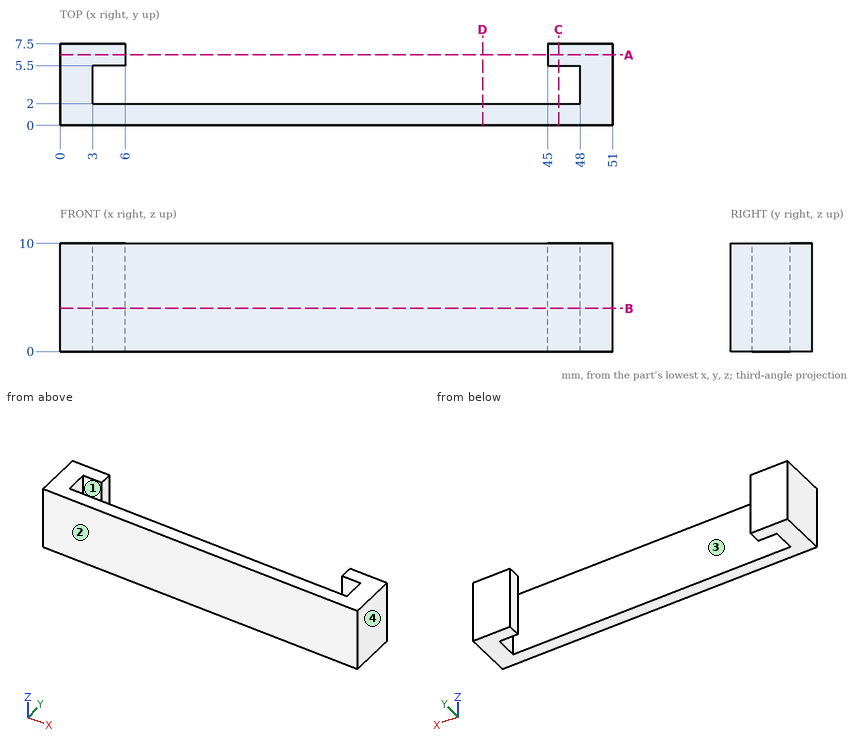
Geometry check sheet. Reference: drawing and pictorial views, mm from the part's lowest x, y, z. Give positions to 0.01 mm unless a question says otherwise; leave off trailing zeros. Order: outer loops, then holes, each group sorted by start corner. A loop starts at its lowest first (then second) coordinate and runs counter-clockwise, first axis right, second up.
1. Thickness scan on L1, parallel to X at y = 3.5, z = 1.25; L2, parallel to Y at x = 46, z = 6.5; L3, parallel to Y at x = 8, z = 6.25. Record the ranges inside material, lowest first.
2. Section check B-B, the plane z = 4. Enter the section's corners in (x, y), and give its area (3 significant figures).
3. Section check A-A, the plane y = 6.5. Enter the section's corners in (x, z).
4. Release check for a two-part mould opening along X. For the marked faces 1, 2, 3 and 4 record: pulls with the +X half, pulls with the -X half, needs draft (parallel to the pull), parting line crosses it, or undercut.
5. Section check C-C, the plane x = 46. Enter the section's corners in (y, z).
6. Section check D-D, the plane x = 39. Enter the section's corners in (y, z).
7. Gauge pin test, flat end, axial feed: pin 1 Ø3 at (x, z) = (38, 1.5) entering from +Y. Record the tip position at first contact, or that the pin passes through.
Values follow:
1. L1: x = 0 to 3, 48 to 51
1. L2: y = 0 to 2, 5.5 to 7.5
1. L3: y = 0 to 2
2. outline: (0, 0) - (51, 0) - (51, 7.5) - (45, 7.5) - (45, 5.5) - (48, 5.5) - (48, 2) - (3, 2) - (3, 5.5) - (6, 5.5) - (6, 7.5) - (0, 7.5) - close
2. area: 147 mm2
3. outline: (0, 0) - (6, 0) - (6, 10) - (0, 10) - close; (45, 0) - (51, 0) - (51, 10) - (45, 10) - close
4. face 1: undercut
4. face 2: needs draft
4. face 3: undercut
4. face 4: pulls with the +X half
5. outline: (0, 0) - (2, 0) - (2, 10) - (0, 10) - close; (5.5, 0) - (7.5, 0) - (7.5, 10) - (5.5, 10) - close
6. outline: (0, 0) - (2, 0) - (2, 10) - (0, 10) - close
7. pin 1: stops at y = 2
